The drawing under review shows one solid part. Ordinate dimensions are in mm from its lowest x, y, z. A direction names the side the tool comes from. Round coordinates to 2 decimals unless told otherwise and drop trailing zeros. Write each loop counter-clockwise with the first axis right and the second up, starting at its lowest first coordinate (ties: lowest second). Pieces come first, ordered by that corner, then holes. Notation, with made-up numbers: (28, 33.5) - (58, 33.5) arc R14 ccw to (58, 49.5) - close; hole circle Ø2 at (79, 6.25). An arc over 180 degrees is marked (long way). One line per question, with ' | ' between items. Start each with the question number.
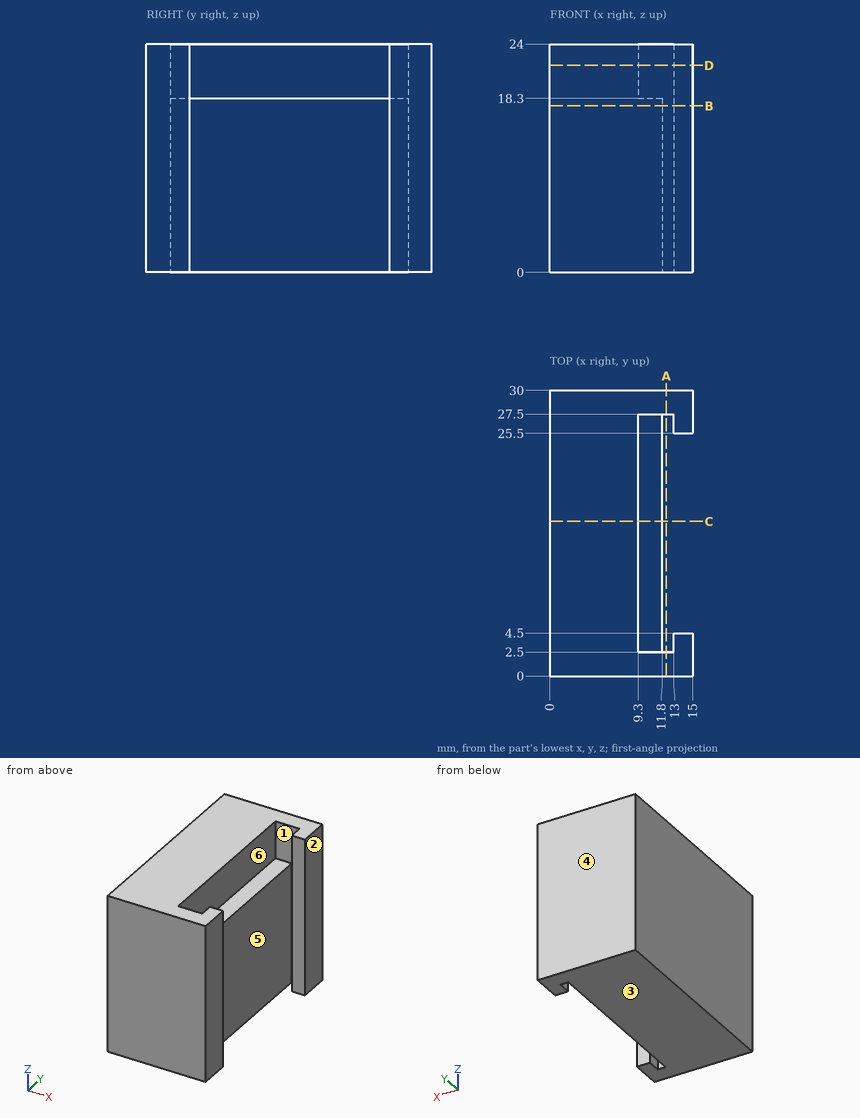
1. The part is to be moulded in two halves that separate along X. For the marked faces 1, 2 and 3, say which applies: pulls with the +X half, pulls with the -X half, needs draft (parallel to the pull), parting line crosses it, or undercut.
2. Machinability: for the marked faces 4, 5 and 6, which of the approach directions +Z, -Z, +X, -X, +Y, -Y give a long, thin tool a straight path to every point of the face, cutting with its end or side? Answer none if there is none.
3. Add section A-A, the plane x = 12.25. Write out the cut boundary in (y, z).
4. Add section B-B, the plane z = 17.5. Write out the cut boundary in (x, y).
5. Wall thickness on line 1 along Y through (x, z) = (13.25, 16.5); line 2 along Y through (x, z) = (10.25, 22); line 3 along X through (y, z) = (12.5, 13): over which ranges is each line inside the solid? List them lowest first. Write a range as [from, to].
6. Add section D-D, the plane z = 21.75. Write out the cut boundary in (x, y).
7. Clearance check with flat-ended pins moving along their axes: P1, Ø0.8, axis at x = 10.5, y = 19.5, coming from the +Z side; P2, Ø3, axis at y = 17.5, z = 21, coming from the +X side. State where each tip first meets the part, or that it passes through.
8. Add section C-C, the plane y = 16.25. Write out the cut boundary in (x, z), then the cut area to 3 significant figures.
Geometry check:
1) face 1: undercut | face 2: pulls with the +X half | face 3: needs draft
2) face 4: +Z, -Z, +X, -X, +Y | face 5: +Z, -Z | face 6: +Z
3) outline: (0, 0) - (2.5, 0) - (2.5, 24) - (0, 24) - close; (27.5, 0) - (30, 0) - (30, 24) - (27.5, 24) - close
4) outline: (0, 0) - (15, 0) - (15, 4.5) - (13, 4.5) - (13, 2.5) - (11.8, 2.5) - (11.8, 27.5) - (13, 27.5) - (13, 25.5) - (15, 25.5) - (15, 30) - (0, 30) - close
5) line 1: y = [0, 4.5], [25.5, 30] | line 2: y = [0, 2.5], [27.5, 30] | line 3: x = [0, 11.8]
6) outline: (0, 0) - (15, 0) - (15, 4.5) - (13, 4.5) - (13, 2.5) - (9.3, 2.5) - (9.3, 27.5) - (13, 27.5) - (13, 25.5) - (15, 25.5) - (15, 30) - (0, 30) - close
7) P1: stops at z = 18.3 | P2: stops at x = 9.3
8) outline: (0, 0) - (11.8, 0) - (11.8, 18.3) - (9.3, 18.3) - (9.3, 24) - (0, 24) - close | area: 269 mm2
